Build history of the part. All positions in model axes, mm. A direction names the side the tool comes from. Round coordinates to 2 decimals unless told otherwise and drop trailing zeros. Write each loop counter-clockwise with the first axis right and the second up, starting at its lowest first coordinate (ties: lowest second). Pieces come first, ordered by that corner, then holes.
Item 1: Band-saw the part on B-B, the plane y = 36.5. Write the cut outline in (x, z), then the cut area to 3 significant figures.
Item 2: Drop flat-ended pins along their axis: pin 1 Ø1.5 at (x, z) = (14.5, 13) entering from -Y; pin 2 Ø10 at (y, z) = (11.5, 6.5) entering from +X; pin 3 Ø2 at (x, z) = (29, 16) entering from +Y. Give the stop position or say it passes through.
Item 3: Mould opens along X. For faces 1 (the cylindrical face through (15.68, 1.97, 11.48)), 2 (the flat face through (3, 32, 7)), 3 (the flat face through (-1.5, 29, 10)), 4 (the flat face through (42, 21, -2)) say: +X half, -X half, draft (parallel to the pull), parting line (faces both ways), or undercut.
Item 4: Wall check: probe 1 along Y at (x, z) = (36.5, -1); probe 2 along Y at (x, z) = (21, -2.35); probe 3 along Y at (x, z) = (5.5, -1.1). Give the ranges that are in metal, low to high.
Item 5: Band-saw the part on C-C, the plane x = 13.5. Write the cut outline in (y, z), then the cut area to 3 significant figures.
Item 6: Band-saw the part on A-A, the plane y = 5.5. Write the cut outline in (x, z).
Item 7: Band-saw the part on D-D, the plane z = 10. Count the separate pieces of the cut face and the enclosed holes in it, then the cut area to 3 significant figures.
Item 8: 3-axis set-ups, long thin cutter, end or side, ignore diameter. For faces 5 (the flat face through (9, 10, 10)), 6 (the flat face through (25, -1, 10)), 7 (the flat face through (0, 19, 5)), 8 (the flat face through (32, 3, 7)): which of +Z, -Z, +X, -X, +Y, -Y reach the whole face in a straight line?
Autodesk Fusion 360 part; units mm, degrees
sketch "Sketch1" plane through (0, 0, 0) normal (0, 0, 1) x (-1, 0, 0)
  line L0 (-42, -42) -> (-42, 0)
  circle A0 centre (-36.5, -36.5) radius 1.7
  circle A1 centre (-36.5, -5.5) radius 1.7
  circle A2 centre (-5.5, -5.5) radius 1.7 construction
  circle A3 centre (-5.5, -36.5) radius 1.7
  line L1 (-5.5, -36.5) -> (-36.5, -36.5) construction
  line L2 (-36.5, -5.5) -> (-5.5, -5.5) construction
  line L3 (-36.5, -36.5) -> (-36.5, -5.5) construction
  circle A4 centre (-21, -21) radius 11.5
  line L4 (0, 0) -> (0, -42)
  line L5 (0, 0) -> (-42, 0)
  line L6 (-5.5, -5.5) -> (-36.5, -36.5) construction
  line L7 (-5.5, -36.5) -> (-5.5, -5.5) construction
  line L8 (-8, -8) -> (-32, -8)
  line L9 (-32, -8) -> (-32, 0)
  line L10 (-8, -8) -> (-8, -32)
  line L11 (-8, -32) -> (0, -32)
  line L12 (0, -42) -> (-42, -42)
  circle A5 centre (-36.5, -5.5) radius 4 construction
  circle A6 centre (-5.5, -36.5) radius 4 construction
  dimension "d1130" = 31
  dimension "d1131" = 31
  dimension "d1132" = 3.4
  dimension "d1173" = 23
  dimension "d1184" = 0
  dimension "d1185" = 0
  dimension "d1186" = 0
  dimension "d1187" = 0
  dimension "d1331" = 42
  dimension "d1332" = 42
  dimension "d1339" = 0
  dimension "d1340" = 0
  dimension "d1341" = 0
  dimension "d1342" = 0
  dimension "d1367" = 0
  dimension "d1368" = 0
  dimension "d1369" = 0
  dimension "d1370" = 0
  dimension "d1450" = 0
  dimension "d1451" = 0
  dimension "d1452" = 0
  dimension "d1453" = 0
  dimension "d1458" = 0
  dimension "d1459" = 0
  dimension "d1460" = 0
  dimension "d1461" = 0
  dimension "d1615" = 0
  dimension "d1616" = 0
  dimension "d1617" = 0
  dimension "d1618" = 0
  dimension "d2598" = 32
  dimension "d2" = 32
  dimension "d4" = 20
  dimension "d181" = 5.5
  dimension "d182" = 8
  dimension "d199" = 0
  dimension "d200" = 0
  dimension "d201" = 0
  dimension "d202" = 0
  dimension "d277" = 8
extrude "Extrude1" add sketch "Sketch1" against normal blind 4
chamfer "Chamfer6" distance 4 angle 45 3 edges at (42, 0, -2) (0, 42, -2) (42, 42, -2)
extrude "Extrude6" add sketch "Sketch1" along normal blind 20 contours L4 L5 L8 L9 L10 L11
sketch "Sketch6" plane through (32, 0, 0) normal (1, 0, 0) x (0, 1, 0)
  line L0 (0, 0) -> (8, 0)
  line L1 (8, 0) -> (8, 20)
  line L2 (8, 20) -> (0, 20)
  line L3 (0, 20) -> (0, 0)
  line L4 (0, 10) -> (-1.5, 10) construction
  line L5 (0, 14.5) -> (-1.5, 13)
  line L6 (-1.5, 13) -> (-1.5, 7)
  line L7 (-1.5, 7) -> (0, 5.5)
  dimension "d7" = 1.5
  dimension "d8" = 6
extrude "Extrude11" add sketch "Sketch6" against normal blind 8 contours L3 L5 L6 L7
extrude "Extrude12" add 1 faces at (24, -0.5, 11) along direction (-1, 0, 0) blind 12 from surface at 12
ref_plane "WorkPlane1" through (0, 0, 8) normal (0.7071, -0.7071, 0) x (0, 0, -1)
mirror "Mirror1" about plane through (0, 0, 8) normal (0.7071, -0.7071, 0) of "Extrude11", "Extrude12"
hole "Hole3" at (18, 8, 10) direction (0, -1, 0) diameter 5.5 depth 19 tip angle 118 counterbore diameter 12 counterbore depth 4
hole "Hole4" at (8, 18, 10) direction (-1, 0, 0) diameter 5.5 depth 12 tip angle 118 counterbore diameter 12 counterbore depth 4
chamfer "Chamfer4" distance 5 angle 45 2 edges at (32, 4, 20) (4, 32, 20)
chamfer "Chamfer7" distance 1.5 angle 45 6 edges at (12, -1.5, 10) (24, -1.5, 10) (-1.5, 12, 10) (-1.5, 24, 10) (0, -1.5, 10) (-1.5, 0, 10)
chamfer "Chamfer8" distance 3 angle 45 1 edges at (8, 8, 10)
equation "d1131 = d1130"
equation "d1332 = d1331"
equation "d2 = d2598"
Results:
1. outline: (0, -4) - (3.8, -4) - (3.8, 0) - (0, 0) - close; (7.2, -4) - (34.8, -4) - (34.8, 0) - (7.2, 0) - close; (38.2, -4) - (42, -4) - (42, 0) - (38.2, 0) - close
1. area: 141 mm2
2. pin 1: stops at y = 0
2. pin 2: stops at x = 32
2. pin 3: stops at y = 8
3. face 1: undercut
3. face 2: draft
3. face 3: -X half
3. face 4: +X half
4. probe 1: y = 0 to 3.8, 7.2 to 34.8, 38.2 to 42
4. probe 2: y = 0 to 9.5, 32.5 to 42
4. probe 3: y = 0 to 34.8, 38.2 to 42
5. outline: (0, -4) - (12.28, -4) - (12.28, 0) - (8, 0) - (8, 6.03) - (4, 6.03) - (4, 13.97) - (8, 13.97) - (8, 20) - (0, 20) - close; (29.72, -4) - (42, -4) - (42, 0) - (29.72, 0) - close
5. area: 227 mm2
6. outline: (-1.5, 7) - (0, 5.5) - (0, -4) - (34.8, -4) - (34.8, 0) - (32, 0) - (32, 15) - (27, 20) - (0, 20) - (0, 14.5) - (-1.5, 13) - close; (38.2, -4) - (42, -4) - (42, 0) - (38.2, 0) - close; hole circle Ø12 at (18, 10)
7. separate pieces: 3
7. enclosed holes: 0
7. area: 366 mm2
8. face 5: +Z, +X, +Y
8. face 6: +Z, -Z, -Y
8. face 7: -X
8. face 8: +Z, +X, +Y, -Y
